Source: three-view drawing plus pictorial views. Frame: mm from the lowest corner of the part. A direction names the side the tool comes from. Give positions to 0.01 mm unless a question says otherwise; leave off trailing zeros. Order: outer loops, then holes, each group sorted by start corner. A loop starts at its lowest first (then second) coordinate and runs counter-clockwise, first axis right, second up.
1) Access query for the marked faces 1 and 2. Directions: +Z, -Z, +X, -X, +Y, -Y. A direction counts if a zero-diameter tool reaches every point of the face in a straight line with its end or side. Return the directions, or none.
2) Section A-A, the plane z = 20.5. Return loops of the section in (x, y), plus the area to 4 significant figures.
3) Material intervals for line 1 (X direction, y = 13, z = 14); line 2 (Z direction, x = 12.5, y = 11); line 3 (Z direction, x = 5.5, y = 6), sorted ascending.
4) First-contact query: P1, Ø4, axis at x = 6, z = 20, coming from the +Y side. Flat tip, straight axial feed; report the tip coordinate or a pass-through.
5) Section B-B, the plane x = 21.75. Return loops of the section in (y, z), plus the area to 3 significant figures.
6) Section D-D, the plane x = 9.75. Return loops of the section in (y, z), plus the area to 4 significant figures.
7) Section C-C, the plane y = 9. Return loops of the section in (x, z).
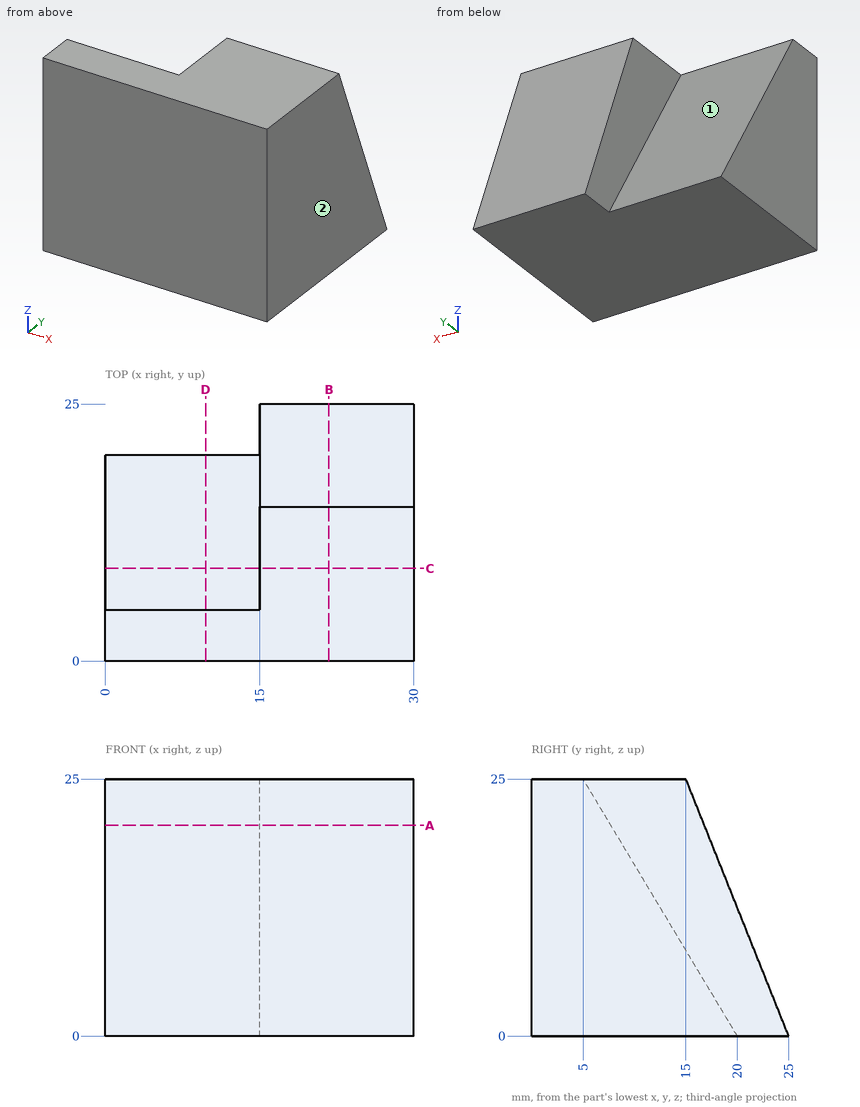
From the geometry:
1. face 1: +Z, -X, +Y
1. face 2: +Z, -Z, +X, +Y, -Y
2. outline: (0, 0) - (30, 0) - (30, 16.8) - (15, 16.8) - (15, 7.7) - (0, 7.7) - close
2. area: 367.5 mm2
3. line 1: x = 15 to 30
3. line 2: z = 0 to 15
3. line 3: z = 0 to 23.33
4. P1: stops at y = 9.2
5. outline: (0, 0) - (25, 0) - (15, 25) - (0, 25) - close
5. area: 500 mm2
6. outline: (0, 0) - (20, 0) - (5, 25) - (0, 25) - close
6. area: 312.5 mm2
7. outline: (0, 0) - (30, 0) - (30, 25) - (15, 25) - (15, 18.33) - (0, 18.33) - close
